For this review, take the finished solid that the model builds, in its own axes (mm). Face numbers are marked on the shaded views. A direction names the side the tool comes from. Round coordinates to 2 decimals unless told otherwise and drop trailing zeros. Order: outer loops, then holes, each group sorted by start corner. A loop starts at its lowest first (then second) coordinate and runs counter-clockwise, first axis right, second up. Notation, with made-up numbers: (63, -6.75) -> (103, -6.75) arc R11 ccw to (103, 12.25) -> close; hole circle Ø6 at (87.5, 9). An arc over 180 degrees is marked (long way). Use a Markdown table: item, result. Add a question column.
1) Consider section B-B (x = -3). State the section outline as (y, z) points, plus the area to 3 significant figures.
2) Draft analysis for pull direction Z (two halves, no side actions). For the marked faces 3, 4, 5 and 6, state which applies: pulls with the +Z half, pulls with the -Z half, needs draft (parallel to the pull), parting line crosses it, or undercut.
3) Machinability: for the marked faces 1 and 2, which of the approach directions +Z, -Z, +X, -X, +Y, -Y give a long, thin tool a straight path to every point of the face, cutting with its end or side? Answer none if there is none.
4) Consider section A-A (x = 16.5). State the section outline as (y, z) points.
5) Wall thickness on line 1 along Y through (x, z) = (16, 0.25); line 2 along X through (y, z) = (-3, -4); line 3 along Z through (x, y) = (14, 1.25): over which ranges is each line inside the solid? List them lowest first. Write a range as [from, to].
6) Clearance check with flat-ended pins moving along their axes: P1, Ø1.5, axis at x = 6, y = 2, coming from the -Z side; P2, Ø4, axis at x = 21, z = -4.5, coming from the -Y side; P3, Ø6, axis at x = 24.5, z = 1.5, coming from the +Y side. State where each tip first meets the part, or that it passes through.
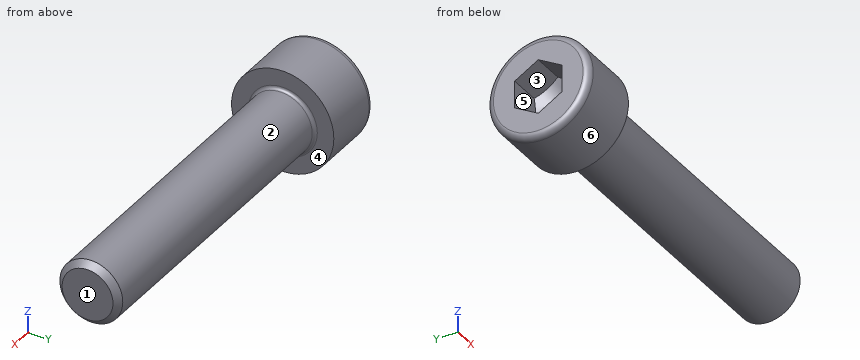
Autodesk Inventor part; units mm, degrees
ref_plane "Work Plane1" through (29, 0, 0) normal (0, -1, 0) x (1, 0, 0)
ref_plane "YZ Plane" through (0, 0, 0) normal (1, 0, 0) x (0, 1, 0)
ref_plane "XZ Plane" through (0, 0, 0) normal (0, 1, 0) x (-1, 0, 0)
sketch "Sketch1" plane through (0, 0, 0) normal (0, 0, 1) x (1, 0, 0)
  line L0 (-2, 0) -> (40, 0)
  line L1 (40, 0) -> (40, 4)
  line L2 (40, 4) -> (3.125, 4)
  line L3 (3.125, 4) -> (2.3581, 4)
  line L4 (2.3581, 4) -> (0, 4)
  line L5 (0, 4) -> (0, 6.5)
  line L6 (0, 6.5) -> (-8, 6.5)
  line L7 (-8, 6.5) -> (-8, 3.4641)
  line L8 (-8, 3.4641) -> (-4, 3.4641)
  line L9 (-4, 3.4641) -> (-2, 0)
  line L10 (-17.6, 0) -> (49.6, 0)
  line L11 (0, -1.3) -> (0, 7.8)
  line L12 (3.125, 4) -> (0, 4) construction
  dimension "d1" = 36.875
  dimension "d2" = 0.7669
  dimension "d3" = 8
  dimension "d4" = 4
  dimension "d5" = 60
  dimension "d6" = 8
  dimension "d7" = 8
  dimension "d8" = 6.9282
  dimension "d9" = 13
  dimension "d26" = 40
revolve "Body" add sketch "Sketch1" angle 360 about axis through (-2, 0, 0) along (1, 0, 0)
sketch "Sketch2" plane through (-8, 0, 0) normal (-1, 0, 0) x (0, 0, 1)
  circle A0 centre (0, 0) radius 3.4641
  line L0 (0, -9.1) -> (0, 9.1)
  line L1 (-9.1, 0) -> (9.1, 0)
  line L2 (3.4641, 0) -> (1.7321, -3)
  line L3 (1.7321, -3) -> (-1.7321, -3)
  line L4 (-1.7321, -3) -> (-3.4641, 0)
  line L5 (-3.4641, 0) -> (-1.7321, 3)
  line L6 (-1.7321, 3) -> (1.7321, 3)
  line L7 (1.7321, 3) -> (3.4641, 0)
extrude "Slot" add sketch "Sketch2" against normal up to next contours L7 A0 | A0 L2 | L6 L0 A0 | A0 L0 L3 | L0 L6 A0 | A0 L3 L0 | L4 A0 | A0 L5
fillet "Fillet1" radius 0.8 1 edges at (-8, -6.5, 0)
thread "Thread"
chamfer "Chamfer1" distance 0.7668 distance2 0.7668 1 edges at (40, -4, 0) measured on face at (40, -0.998, -0.8842)
ref_plane "Work Plane1" through (29, 0, 0) normal (0, -1, 0) x (1, 0, 0)
fillet "Fillet2" radius 0.4 1 edges at (0, -4, 0)
equation "\"d3\" = KOH"
equation "\"d4\" = INTI"
equation "\"d6\" = GD"
equation "\"d7\" = BDM"
equation "\"d8\" = 1.1547 * SW"
equation "\"d9\" = KOD"
equation "\"d30\" = R"
equation "\"d17\" = RR"
equation "\"d15\" = -0.5 * SPD + 0.5 * GD"
equation "\"d16\" = GUL"
equation "\"GD\" = NND"
equation "\"NLG\" = 25"
equation "\"GEL\" = 21.875"
equation "\"KOD\" = 13"
equation "\"KOH\" = 8"
equation "\"INTI\" = 4"
equation "\"GAL\" = 0.61345 * PTC"
equation "\"GUL\" = 0.61345 * PTC"
equation "\"BDM\" = NND"
equation "\"SW\" = 6"
equation "\"RR\" = 0.8"
equation "\"SPD\" = NND - 1.2269 * PTC"
equation "\"R\" = 0.4"
equation "\"TOA\" = 30deg"
equation "\"GD1\" = THREADDIA - 1.2269 * PTC"
equation "\"THREADDIA\" = 8"
equation "\"FAWI\" = 45deg"
equation "\"ANG\" = 120deg"
equation "\"PTC\" = 1.25"
equation "\"NND\" = 8"
equation "\"E0\" = 1.155 * SW"
properties part number "Allen Key 8x40mm" material "Steel, Mild"
Results list:
| question | item | result |
|---|---|---|
| 1 | outline | circle Ø13 at (0, 0); hole circle Ø3.46 at (0, 0) |
| 1 | area | 123 mm2 |
| 2 | face 3 | undercut |
| 2 | face 4 | needs draft |
| 2 | face 5 | undercut |
| 2 | face 6 | parting line crosses it |
| 3 | face 1 | +Z, -Z, +X, +Y, -Y |
| 3 | face 2 | +X |
| 4 | outline | circle Ø8 at (0, 0) |
| 5 | line 1 | [-3.99, 3.99] |
| 5 | line 2 | [-8, 0] |
| 5 | line 3 | [-3.8, 3.8] |
| 6 | P1 | z = -3.8 |
| 6 | P2 | y = -3.12 |
| 6 | P3 | y = 4 |
